Input: dimensioned drawing with shaded views. Units: mm. Origin: part minimum x, y, z. A direction names the side the tool comes from. Round coordinates to 2 decimals unless told otherwise and drop trailing zeros. Order: outer loops, then holes, each group sorted by start corner. A loop starts at its lowest first (then second) coordinate and runs counter-clockwise, first axis right, second up.
Item 1: Cut plane D-D on z = 7. Output: boundary loops of the cut face in (x, y).
Item 2: Reachability of the marked faces 1, 2 and 3 from +Z, -Z, +X, -X, +Y, -Y: full face, straight path, thin tool, end or side. Return the list, or none.
Item 3: Line query: L1, parallel to X at y = 1.85, z = 4; L2, parallel to Z at x = 7.5, y = 1.85; L3, parallel to Z at x = 2.25, y = 0.55. Output: solid intervals per line, ascending.
Item 4: Cut plane A-A on z = 4. Output: boundary loops of the cut face in (x, y).
Item 5: Cut plane B-B on y = 0.5. Output: boundary loops of the cut face in (x, z), then the cut area to 3 significant figures.
Item 6: Cut plane C-C on x = 7.5. Output: boundary loops of the cut face in (y, z).
Item 7: Mould query, pull axis X, two halves, no side actions, for the marked faces 4, 5 and 6. Classes: released by +X, released by -X, zero draft, split by the parting line, or undercut.
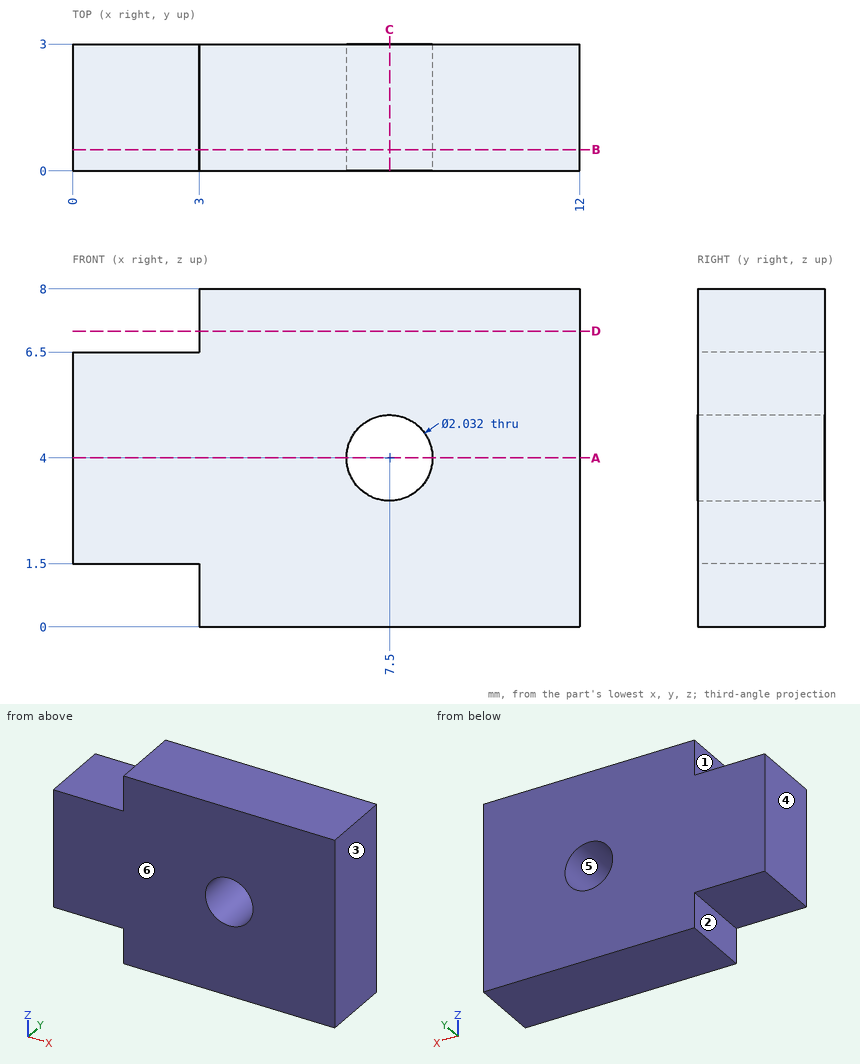
From the geometry:
1. outline: (3, 0) - (12, 0) - (12, 3) - (3, 3) - close
2. face 1: +Z, -X, +Y, -Y
2. face 2: -Z, -X, +Y, -Y
2. face 3: +Z, -Z, +X, +Y, -Y
3. L1: x = 0 to 6.48, 8.52 to 12
3. L2: z = 0 to 2.98, 5.02 to 8
3. L3: z = 1.5 to 6.5
4. outline: (0, 0) - (6.48, 0) - (6.48, 3) - (0, 3) - close; (8.52, 0) - (12, 0) - (12, 3) - (8.52, 3) - close
5. outline: (0, 1.5) - (3, 1.5) - (3, 0) - (12, 0) - (12, 8) - (3, 8) - (3, 6.5) - (0, 6.5) - close; hole circle Ø2.03 at (7.5, 4)
5. area: 83.8 mm2
6. outline: (0, 0) - (3, 0) - (3, 2.98) - (0, 2.98) - close; (0, 5.02) - (3, 5.02) - (3, 8) - (0, 8) - close
7. face 4: released by -X
7. face 5: undercut
7. face 6: zero draft
